The model under review builds one solid part; all positions refer to its coordinate system, in mm. A direction names the side the tool comes from. Coordinates: 2 decimals unless noted, no trailing zeros. Order: outer loops, then holes, each group sorted by start corner. A loop starts at its lowest first (then second) coordinate and runs counter-clockwise, first axis right, second up. Notation, with made-up numbers: M 32.5,86 L 71.5,86 A20 ccw 71.5,96 Z; hole C 10,-18.75 d6. An arc over 180 degrees is marked long. One line per item, written item: value.
```python
from build123d import *

# Parameters (mm, degrees)
SKETCH1_W           = 42
SKETCH1_H           = 7
BOSS_EXTRUDE1_DEPTH = 3
SKETCH3_W           = 5
SKETCH3_H           = 7
BOSS_EXTRUDE2_DEPTH = 7
CUT_EXTRUDE1_DEPTH  = 3
CUT_EXTRUDE2_REACH  = 42.758
SKETCH5_R           = 1.65


with BuildPart() as part:
    # Sketch1 → Boss-Extrude1 (new body)
    with BuildSketch(Plane(origin=(0, 0, 0), x_dir=(1, 0, 0), z_dir=(0, 1, 0))):
        Rectangle(SKETCH1_W, SKETCH1_H)
    boss_extrude1 = extrude(amount=-BOSS_EXTRUDE1_DEPTH)

    # Sketch3 → Boss-Extrude2 (add)
    with BuildSketch(Plane(origin=(0, 0, 0), x_dir=(1, 0, 0), z_dir=(0, 1, 0))):
        with Locations((-18.5, 0)):
            Rectangle(SKETCH3_W, SKETCH3_H)
    boss_extrude2 = extrude(amount=BOSS_EXTRUDE2_DEPTH)

    # Sketch4 → Cut-Extrude1 (cut)
    with BuildSketch(Plane(origin=(-16, 0, 0), x_dir=(0, 0, -1), z_dir=(1, 0, 0))):
        Polygon((1.443375673, 6), (-1.443375673, 6), (-2.886751346, 3.5), (-1.443375673, 1), (1.443375673, 1), (2.886751346, 3.5), align=None)
    cut_extrude1 = extrude(amount=-CUT_EXTRUDE1_DEPTH, mode=Mode.SUBTRACT)

    # Sketch5 → Cut-Extrude2 (cut, up to next)
    with BuildSketch(Plane(origin=(-19, 0, 0), x_dir=(0, 0, -1), z_dir=(1, 0, 0)), mode=Mode.PRIVATE) as cut_extrude2_sk1:
        with Locations((0, 3.5)):
            Circle(SKETCH5_R)
    cut_extrude2_tool1 = extrude(cut_extrude2_sk1.sketch, amount=-CUT_EXTRUDE2_REACH, mode=Mode.PRIVATE) & part.part
    cut_extrude2 = cut_extrude2_tool1.solids().sort_by_distance((-19, 3.5, 0))[0]
    add(cut_extrude2, mode=Mode.SUBTRACT)

    # Mirror3: Boss-Extrude1 across plane
    add(boss_extrude1.mirror(Plane.ZX.offset(3.5)))

    # Mirror4: Boss-Extrude2, Cut-Extrude1, Cut-Extrude2 across plane
    add(boss_extrude2.mirror(Plane(origin=(0, 0, 0), x_dir=(0, 0, 1), z_dir=(1, 0, 0))))
    add(cut_extrude1.mirror(Plane(origin=(0, 0, 0), x_dir=(0, 0, 1), z_dir=(1, 0, 0))), mode=Mode.SUBTRACT)
    add(cut_extrude2.mirror(Plane(origin=(0, 0, 0), x_dir=(0, 0, 1), z_dir=(1, 0, 0))), mode=Mode.SUBTRACT)


solid = part.part
```
(1) We need section C-C, the plane z = 0. State the section outline as (x, y) points.
Geometry results:
outline: M -21,-3 L 21,-3 L 21,1.85 L 19,1.85 L 19,1 L 16,1 L 16,0 L -16,0 L -16,1 L -19,1 L -19,1.85 L -21,1.85 Z; M -21,5.15 L -19,5.15 L -19,6 L -16,6 L -16,7 L 16,7 L 16,6 L 19,6 L 19,5.15 L 21,5.15 L 21,10 L -21,10 Z
(2) We need section A-A, the plane x = 10.5. State the section outline as (y, z) points.
Geometry results:
outline: M -3,-3.5 L 0,-3.5 L 0,3.5 L -3,3.5 Z; M 7,-3.5 L 10,-3.5 L 10,3.5 L 7,3.5 Z
(3) We need section D-D, the plane z = 2.5. State the section outline as (x, y) points, plus the area to 3 significant figures.
Geometry results:
outline: M -21,-3 L 21,-3 L 21,10 L -21,10 Z; hole M -19,2.83 L -16,2.83 L -16,0 L 16,0 L 16,2.83 L 19,2.83 L 19,4.17 L 16,4.17 L 16,7 L -16,7 L -16,4.17 L -19,4.17 Z
area: 314 mm2
(4) Mouldability with a two-part tool opening along Y and no side actions: class faces 4 (the flat face through (17, 6, 0)), 5 (the flat face through (21, 2, 1)), 6 (the flat face through (0, 10, 0)), 7 (the flat face through (-17, 6, 0)) as +Y half, -Y half, draft (parallel to the pull), parting line (faces both ways), or undercut.
Geometry results:
face 4: undercut
face 5: draft
face 6: +Y half
face 7: undercut
(5) For L1, parallel to Y at x = 20, z = 0; L2, parallel to Y at x = 8, z = -2.25; L3, parallel to X at y = 4, z = 3, list the stretches that pass through material, from the lowest coordinate up.
Geometry results:
L1: y = -3 to 1.85, 5.15 to 10
L2: y = -3 to 0, 7 to 10
L3: x = -21 to -16, 16 to 21
(6) Tool access review of faces 1 (the flat face through (17, 1, 0)), 2 (the flat face through (16, 1.9, 2.4)), 3 (the flat face through (0, -1, 3.5)): name each direction out of +Z, -Z, +X, -X, +Y, -Y from which nothing blocks a thin tool from reaching the whole face with its end or side.
Geometry results:
face 1: none
face 2: +Z, -Z
face 3: +Z, +X, -X, +Y, -Y
(7) We need section B-B, the plane y = 6.5. State the section outline as (x, z) points, plus the area to 3 significant figures.
Geometry results:
outline: M -21,-3.5 L -16,-3.5 L -16,3.5 L -21,3.5 Z; M 16,-3.5 L 21,-3.5 L 21,3.5 L 16,3.5 Z
area: 70.0 mm2
